The drawing under review shows one solid part. Ordinate dimensions are in mm from its lowest x, y, z. A direction names the side the tool comes from. Give positions to 0.01 mm unless a question says otherwise; leave off trailing zeros. Loops run counter-clockwise (first coordinate to the right, second up) from the corner with the lowest first, then second, coordinate; pieces in that order, holes last. Notation, with made-up numbers: M 47,88.5 L 81,88.5 A27 cw 81,117.5 Z; hole C -24,-15 d11. An arc over 180 degrees is marked long. One line per item, written item: value. Start each with the question number.
Q1. Mouldability with a two-part tool opening along X and no side actions: class the marked faces 1, 2 and 3 as released by +X, released by -X, zero draft, split by the parting line, or undercut.
Q2. We need section D-D on y = 221. Write out the cut boundary in (x, z), plus the area to 3 significant figures.
Q3. For the marked faces 4 and 5, list the 3-axis set-ups (+Z, -Z, +X, -X, +Y, -Y) from which the entire face can be reached by the end or side of a thin tool; tool diameter is ignored.
Q4. We need section A-A on y = 113. Write out the cut boundary in (x, z).
Q5. To check wall thickness, follow line 1 along X through (y, z) = (211.5, 50); line 2 along Y through (x, z) = (168, 6); line 3 along Z through (x, y) = (328.5, 26.5). State the ranges of each line that lie inside material, in increasing order. Write a range as from..to.
Q6. We need section C-C on z = 60. Write out the cut boundary in (x, y), plus the area to 3 significant figures.
Q7. We need section B-B on x = 116. Write out the cut boundary in (y, z), plus the area to 3 significant figures.
Q8. For pin 1 (5 mm diameter, centred on y = 197.5, z = 39.5, fed in from -X); pin 2 (1 mm diameter, centred on y = 153.5, z = 67, fed in from +X); pin 3 (12 mm diameter, centred on x = 89, z = 55, fed in from -Y), all flat-tipped, find the tip position at first contact; note any pin that passes through.
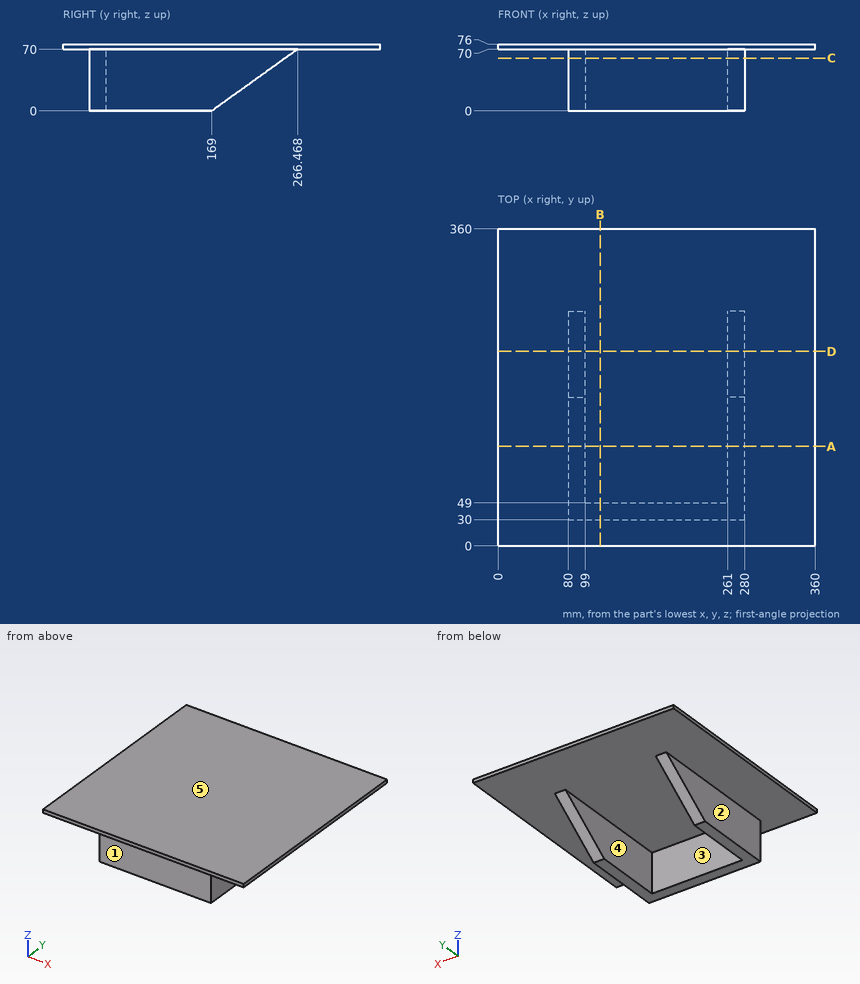
Solved:
1. face 1: zero draft
1. face 2: released by -X
1. face 3: undercut
2. outline: M 0,70 L 80,70 L 80,37.35 L 99,37.35 L 99,70 L 261,70 L 261,37.35 L 280,37.35 L 280,70 L 360,70 L 360,76 L 0,76 Z
2. area: 3,400 mm2
3. face 4: -Z, +Y
3. face 5: +Z, +X, -X, +Y, -Y
4. outline: M 0,70 L 80,70 L 80,0 L 99,0 L 99,70 L 261,70 L 261,0 L 280,0 L 280,70 L 360,70 L 360,76 L 0,76 Z
5. line 1: 80..99, 261..280
5. line 2: 30..49
5. line 3: 70..76
6. outline: M 80,30 L 280,30 L 280,252.54 L 261,252.54 L 261,49 L 99,49 L 99,252.54 L 80,252.54 Z
6. area: 11,500 mm2
7. outline: M 0,70 L 30,70 L 30,0 L 49,0 L 49,70 L 360,70 L 360,76 L 0,76 Z
7. area: 3,490 mm2
8. pin 1: x = 80
8. pin 2: x = 280
8. pin 3: y = 30
